Can you work these out from the model? Positions are in its coordinate system, mm. Face numbers are marked on the shaded views. A direction names the side the tool comes from. Give positions to 0.01 mm unless a question says otherwise; leave off trailing zeros. Loops run counter-clockwise (first coordinate to the right, second up) from the corner with the lowest first, then second, coordinate; pieces in that order, holes last. Notation, with made-up numbers: (89, 68.25) - (123, 68.25) arc R28 ccw to (123, 89.25) - close; hole circle Ø2 at (84.5, -3). An arc over 180 degrees is marked (long way). Use a Markdown table: item, result. Add a question column.
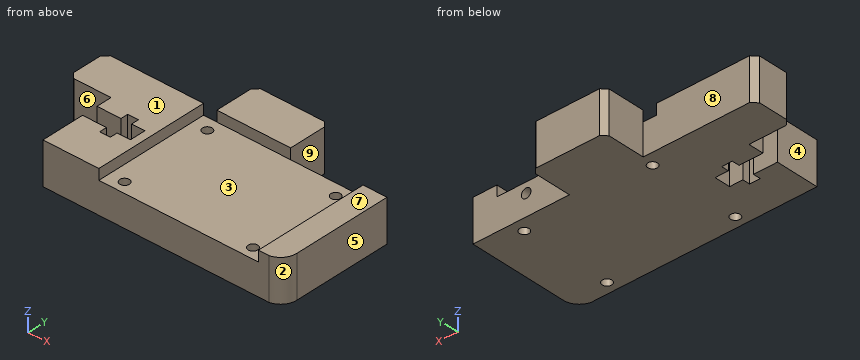
```python
from build123d import *

# Parameters (mm, degrees)
SKETCH002_W  = 30
SKETCH002_H  = 21.7
PAD002_DEPTH = 2
SKETCH001_R  = 0.9
PAD001_DEPTH = 10
PAD_DEPTH    = 7.9
SKETCH005_R  = 0.9
POCKET_DEPTH = 12.5


with BuildPart() as pcb_placement_puncher:
    # Sketch002 → Pad002 (new body)
    with BuildSketch(Plane.XY.offset(7.9)):
        with Locations((7, -5.35)):
            Rectangle(SKETCH002_W, SKETCH002_H)
    extrude(amount=-PAD002_DEPTH)


with BuildPart() as holes_for_pcb_puncher:
    # Sketch001 → Pad001 (new body)
    with BuildSketch(Plane.XY):
        with Locations((-5.09, 3.09)):
            Circle(SKETCH001_R)
        with Locations((19.04, 3.09)):
            Circle(SKETCH001_R)
        with Locations((19.04, -14.06)):
            Circle(SKETCH001_R)
        with Locations((-5.09, -14.06)):
            Circle(SKETCH001_R)
    extrude(amount=PAD001_DEPTH)


with BuildPart() as i3b1_31_with_ir_probe_pcb_holder:
    # Sketch → Pad (new body)
    with BuildSketch(Plane.XY):
        with BuildLine():
            Line((-5.5, 5.5), (-5.5, 12.56))
            Line((-5.5, 12.56), (-4.56, 13.5))
            Line((-4.56, 13.5), (7.44, 13.5))
            Line((7.44, 13.5), (8.38, 12.56))
            Line((8.38, 12.56), (8.38, 5.5))
            Line((8.38, 5.5), (26.5, 5.5))
            Line((26.5, 5.5), (26.5, -13.204915))
            ThreePointArc((24, -16.2), (25.792868, -15.15559), (26.5, -13.204915))
            Line((24, -16.2), (-18.5, -16.2))
            Line((-18.5, -16.2), (-18.5, -8))
            Line((-18.5, -8), (-14, -8))
            Line((-14, -8), (-14, -9.4))
            Line((-14, -9.4), (-12, -9.4))
            Line((-12, -9.4), (-12, -8))
            Line((-12, -8), (-9.5, -8))
            Line((-9.5, -8), (-9.5, -5))
            Line((-9.5, -5), (-12, -5))
            Line((-12, -5), (-12, -3.6))
            Line((-12, -3.6), (-14, -3.6))
            Line((-14, -3.6), (-14, -5))
            Line((-14, -5), (-18.5, -5))
            Line((-18.5, -5), (-18.5, -2.1))
            Line((-18.5, -2.1), (-25.5, -2.1))
            Line((-25.5, -2.1), (-26.5, -1.1))
            Line((-26.5, -1.1), (-26.5, 4.5))
            Line((-26.5, 4.5), (-25.5, 5.5))
            Line((-25.5, 5.5), (-5.5, 5.5))
        make_face()
    extrude(amount=PAD_DEPTH)

    # Cut: cut Holes for PCB Puncher
    add(holes_for_pcb_puncher.part, mode=Mode.SUBTRACT)

    # Cut001: cut PCB Placement Puncher
    add(pcb_placement_puncher.part, mode=Mode.SUBTRACT)

    # Sketch005 → Pocket (cut)
    with BuildSketch(Plane(origin=(0, 5.5, 0), x_dir=(-1, 0, 0), z_dir=(0, 1, 0))):
        with Locations((-16.5, 4)):
            Circle(SKETCH005_R)
    extrude(amount=-POCKET_DEPTH, mode=Mode.SUBTRACT)


solid = i3b1_31_with_ir_probe_pcb_holder.part
```
1. Suppose I cut it at D-D (y = -11.25). List the corners of the cut face in (x, z) for me, and give its area (4 significant figures).
2. Suppose I cut it at A-A (y = 3.09). List the corners of the cut face in (x, z) for me.
3. On a 3-axis mill with a long thin cutter (end or side, diameter ignored), from which of +Z, -Z, +X, -X, +Y, -Y can I reach the whole of each face in a straight line? I mean the marked faces 5, 6, 7, 8 and 9. Say none if no direction works.
4. If we mould it in two halves opening along X, with no side actions, what happens to the marked faces 1, 2, 3 and 4? For each: released by +X, released by -X, zero draft, split by the parting line, or undercut.
5. Suppose I cut it at C-C (x = 0). List the corners of the cut face in (y, z) for me, and give its area (3 significant figures).
6. Suppose I cut it at B-B (z = 0.75). State how many separate pieces and enclosed holes the cut face has, and give its area (3 significant figures).
7. Please list where these lines run through material, in increasing order: line 1 along X through (y, z) = (3.09, 2.6); line 2 along X through (y, z) = (2.5, 3.75); line 3 along Y through (x, z) = (-5.09, 2.65). Write a range as [from, to].
8. Will these pins go through, and if not, where does the flat tip stop? P1, Ø0.6, axis at y = -2.5, z = 6.5, coming from the -X side; P2, Ø0.6, axis at x = -1, z = 7.5, coming from the -Y side; P3, Ø2, axis at y = 10, z = 4.5, coming from the -X side.
Results below:
| question | item | result |
|---|---|---|
| 1 | outline | (-18.5, 0) - (26.5, 0) - (26.5, 7.9) - (22, 7.9) - (22, 5.9) - (-8, 5.9) - (-8, 7.9) - (-18.5, 7.9) - close |
| 1 | area | 295.5 mm² |
| 2 | outline | (-26.5, 0) - (-5.99, 0) - (-5.99, 5.9) - (-8, 5.9) - (-8, 7.9) - (-26.5, 7.9) - close; (-4.19, 0) - (18.14, 0) - (18.14, 5.9) - (-4.19, 5.9) - close; (19.94, 0) - (26.5, 0) - (26.5, 7.9) - (22, 7.9) - (22, 5.9) - (19.94, 5.9) - close; hole circle Ø1.8 at (16.5, 4) |
| 3 | face 5 | +Z, -Z, +X, +Y, -Y |
| 3 | face 6 | +Z, -Z, -X, -Y |
| 3 | face 7 | +Z, +X, -X, +Y, -Y |
| 3 | face 8 | +Z, -Z, -X, +Y |
| 3 | face 9 | +Z, -Z, +X, +Y |
| 4 | face 1 | zero draft |
| 4 | face 2 | released by +X |
| 4 | face 3 | undercut |
| 4 | face 4 | released by -X |
| 5 | outline | (-16.2, 0) - (13.5, 0) - (13.5, 7.9) - (5.5, 7.9) - (5.5, 5.9) - (-16.2, 5.9) - close |
| 5 | area | 191 mm² |
| 6 | separate pieces | 1 |
| 6 | enclosed holes | 4 |
| 6 | area | 1,100 mm² |
| 7 | line 1 | [-26.5, -5.99], [-4.19, 18.14], [19.94, 26.5] |
| 7 | line 2 | [-26.5, -5.77], [-4.41, 15.64], [17.36, 18.36], [19.72, 26.5] |
| 7 | line 3 | [-16.2, -14.96], [-13.16, 2.19], [3.99, 12.97] |
| 8 | P1 | x = -18.5 |
| 8 | P2 | y = 5.5 |
| 8 | P3 | x = -5.5 |
